Read the model definition and answer for the solid it produces. Units are mm, in the model's axes. Face numbers are marked on the shaded views. A direction names the side the tool comes from. Coordinates: 2 decimals unless noted, no trailing zeros. Order: outer loops, then holes, each group sorted by start corner. A loop starts at its lowest first (then second) coordinate and runs counter-clockwise, first axis right, second up. Notation, with made-up numbers: (21.5, 49.25) -> (49.5, 49.25) arc R12 ccw to (49.5, 66.25) -> close; hole circle Ø8 at (10.25, 66.25). An arc over 180 degrees is marked (long way). Answer as a JSON object with one key per item and string values. Group by question number.
1) Given pin 1 (1.1 mm diameter, centred on y = -1, z = 46.5, fed in from -X); pin 2 (10 mm diameter, centred on x = 0.5, y = -8.5, fed in from +Z); pin 3 (8 mm diameter, centred on y = -7, z = 18.5, fed in from -X); pin 4 (2 mm diameter, centred on x = -5, z = 33.5, fed in from -Y), each flat-ended and moving along its own axis, determine where each tip first touches the part or whether it passes through.
2) Section B-B on z = 18.5 is taken. Determine the outline of the cut face in (x, y).
3) Consider L1, parallel to Z at x = 11.5, y = 5; L2, parallel to Z at x = -0.5, y = 4.5; L3, parallel to Y at x = -6, z = 1. Determine where each line is inside the solid, lowest interval first.
4) A tool of negligible diameter and unlimited length cuts with its end or side. For the marked faces 1, 2 and 3, from which of +Z, -Z, +X, -X, +Y, -Y can it reach the whole face along a straight path? Write none if from no direction.
5) Section A-A on y = 0 is taken. Determine the outline of the cut face in (x, z), and give its area (3 significant figures).
6) Section C-C on z = -6 is taken. Determine the outline of the cut face in (x, y).
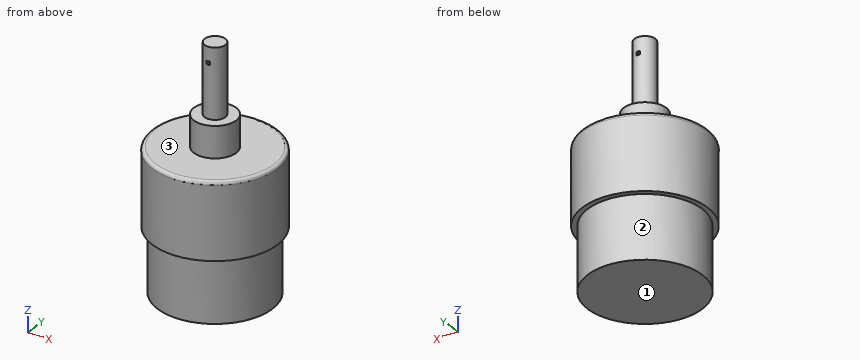
from build123d import *

# Parameters (mm, degrees)
SKETCH1_R           = 18
BOSS_EXTRUDE1_DEPTH = 22
SKETCH2_R           = 6.1
BOSS_EXTRUDE2_DEPTH = 9
SKETCH3_R           = 3
BOSS_EXTRUDE3_DEPTH = 20
SKETCH4_R           = 16.5
BOSS_EXTRUDE4_DEPTH = 18.2
FILLET1_R           = 1
CUT_EXTRUDE1_START  = -4
SKETCH5_W           = 1
SKETCH5_H           = 9.640702938
CUT_EXTRUDE1_DEPTH  = 1


with BuildPart() as part:
    # Sketch1 → Boss-Extrude1 (new body)
    with BuildSketch(Plane.XY):
        Circle(SKETCH1_R)
    extrude(amount=BOSS_EXTRUDE1_DEPTH)

    # Sketch2 → Boss-Extrude2 (add)
    with BuildSketch(Plane.XY.offset(22)):
        Circle(SKETCH2_R)
    extrude(amount=BOSS_EXTRUDE2_DEPTH)

    # Sketch3 → Boss-Extrude3 (add)
    with BuildSketch(Plane.XY.offset(31)):
        Circle(SKETCH3_R)
    extrude(amount=BOSS_EXTRUDE3_DEPTH)

    # Sketch4 → Boss-Extrude4 (add)
    with BuildSketch(Plane(origin=(0, 0, 0), x_dir=(-1, 0, 0), z_dir=(0, 0, -1))):
        with Locations(Location((0, 0, 0), (0, 0, 180))):
            Circle(SKETCH4_R)
    extrude(amount=BOSS_EXTRUDE4_DEPTH)

    # Fillet1
    fillet1_edges = [part.edges().sort_by_distance(p)[0] for p in [
        (-18, 0, 22),
    ]]
    fillet(fillet1_edges, radius=FILLET1_R)

    # Sketch5 → Cut-Extrude1 (cut)
    with BuildSketch(Plane.XY.offset(51).offset(CUT_EXTRUDE1_START)):
        Rectangle(SKETCH5_W, SKETCH5_H)
    extrude(amount=-CUT_EXTRUDE1_DEPTH, mode=Mode.SUBTRACT)


solid = part.part
Worked answers:
{
 "1": {"pin 1": "stops at x = -2.97", "pin 2": "stops at z = 31", "pin 3": "stops at x = -17.75", "pin 4": "passes through"},
 "2": {"outline": "circle Ø36 at (0, 0)"},
 "3": {"L1": "z = -18.2 to 22", "L2": "z = -18.2 to 31", "L3": "y = -16.97 to 16.97"},
 "4": {"face 1": "-Z, +X, -X, +Y, -Y", "face 2": "-Z", "face 3": "+Z"},
 "5": {"outline": "(-18, 0) -> (-16.5, 0) -> (-16.5, -18.2) -> (16.5, -18.2) -> (16.5, 0) -> (18, 0) -> (18, 21) arc R1 ccw to (17, 22) -> (6.1, 22) -> (6.1, 31) -> (3, 31) -> (3, 51) -> (-3, 51) -> (-3, 31) -> (-6.1, 31) -> (-6.1, 22) -> (-17, 22) arc R1 ccw to (-18, 21) -> close; hole (-0.5, 46) -> (0.5, 46) -> (0.5, 47) -> (-0.5, 47) -> close", "area": "1,620 mm²"},
 "6": {"outline": "circle Ø33 at (0, 0)"}
}
